```python
from build123d import *

# Parameters (mm, degrees)
SKETCH1_W                    = 812.8
SKETCH1_H                    = 78.232
BOSS_EXTRUDE1_DEPTH          = 3.175
EDGE_FLANGE1_STRIP_W         = 14.224
EDGE_FLANGE1_STRIP_H         = 3.175
EDGE_FLANGE1_STRIP_CUT_DEPTH = 812.8
EDGE_FLANGE1_DEPTH           = 812.8
EDGE_FLANGE2_STRIP_W         = 14.224
EDGE_FLANGE2_STRIP_H         = 3.175
EDGE_FLANGE2_STRIP_CUT_DEPTH = 812.8
EDGE_FLANGE2_DEPTH           = 812.8
SKETCH9_R                    = 2.667
CUT_EXTRUDE1_DEPTH           = 818.620012948
CHAMFER1_SIZE                = 3.175
SKETCH12_R                   = 1.27
CUT_EXTRUDE4_DEPTH           = 818.20071162
SKETCH15_W                   = 812.8
SKETCH15_H                   = 50.8
BOSS_EXTRUDE2_DEPTH          = 3.175
SKETCH16_W                   = 814.386282527
SKETCH16_H                   = 36.576
BOSS_EXTRUDE3_DEPTH          = 3.175


# Sheet-metal steps are written as plain solids
with BuildPart() as part:
    # Sketch1 → Boss-Extrude1 (new body)
    with BuildSketch(Plane(origin=(0, 0, 0), x_dir=(1, 0, 0), z_dir=(0, 1, 0))):
        with Locations((406.4, 39.116)):
            Rectangle(SKETCH1_W, SKETCH1_H)
    extrude(amount=BOSS_EXTRUDE1_DEPTH)

    # Edge-Flange1 strip (across the edge) → Edge-Flange1 strip cut (cut)
    with BuildSketch(Plane(origin=(812.8, 3.175, -78.232), x_dir=(0, 0, 1), z_dir=(-1, 0, 0))):
        with Locations((-6.35, -1.5875)):
            Rectangle(EDGE_FLANGE1_STRIP_W, EDGE_FLANGE1_STRIP_H)
    extrude(amount=EDGE_FLANGE1_STRIP_CUT_DEPTH, mode=Mode.SUBTRACT)

    # Edge-Flange1 section (across the edge) → Edge-Flange1 (add)
    with BuildSketch(Plane(origin=(812.8, 3.175, -78.232), x_dir=(0, 0, 1), z_dir=(-1, 0, 0))):
        with BuildLine():
            Line((-3.175, 0.762), (-3.175, 23.368))
            Line((-3.175, 23.368), (0, 23.368))
            Line((0, 23.368), (0, 0.762))
            ThreePointArc((0, 0.762), (0.223184633, 0.223184633), (0.762, 0))
            Line((0.762, 0), (0.762, -3.175))
            ThreePointArc((0.762, -3.175), (-2.021879398, -2.021879398), (-3.175, 0.762))
        make_face()
    extrude(amount=EDGE_FLANGE1_DEPTH)

    # Edge-Flange2 strip (across the edge) → Edge-Flange2 strip cut (cut)
    with BuildSketch(Plane(origin=(0, 3.175, 0), x_dir=(0, 0, -1), z_dir=(1, 0, 0))):
        with Locations((-6.35, -1.5875)):
            Rectangle(EDGE_FLANGE2_STRIP_W, EDGE_FLANGE2_STRIP_H)
    extrude(amount=EDGE_FLANGE2_STRIP_CUT_DEPTH, mode=Mode.SUBTRACT)

    # Edge-Flange2 section (across the edge) → Edge-Flange2 (add)
    with BuildSketch(Plane(origin=(0, 3.175, 0), x_dir=(0, 0, -1), z_dir=(1, 0, 0))):
        with BuildLine():
            Line((-3.175, 0.762), (-3.175, 23.368))
            Line((-3.175, 23.368), (0, 23.368))
            Line((0, 23.368), (0, 0.762))
            ThreePointArc((0, 0.762), (0.223184633, 0.223184633), (0.762, 0))
            Line((0.762, 0), (0.762, -3.175))
            ThreePointArc((0.762, -3.175), (-2.021879398, -2.021879398), (-3.175, 0.762))
        make_face()
    extrude(amount=EDGE_FLANGE2_DEPTH)

    # Sketch9 → Cut-Extrude1 (cut, through all)
    with BuildSketch(Plane.XY.offset(3.175)):
        with Locations((806.45, 16.637)):
            Circle(SKETCH9_R)
    extrude(amount=-CUT_EXTRUDE1_DEPTH, mode=Mode.SUBTRACT)

    # Chamfer1
    chamfer1_edges = [part.edges().sort_by_distance(p)[0] for p in [
        (812.8, 26.543, -79.8195),
        (0, 26.543, -79.8195),
        (0, 26.543, 1.5875),
        (812.8, 26.543, 1.5875),
    ]]
    chamfer(chamfer1_edges, length=CHAMFER1_SIZE)

    # Sketch12 → Cut-Extrude4 (cut, through all)
    with BuildSketch(Plane(origin=(0, 3.175, 0), x_dir=(1, 0, 0), z_dir=(0, 1, 0))):
        with Locations(Location((127, 72.39, 0), (0, 0, 270))):
            Circle(SKETCH12_R)
        with Locations(Location((228.6, 72.39, 0), (0, 0, 270))):
            Circle(SKETCH12_R)
        with Locations(Location((228.6, 5.842, 0), (0, 0, 270))):
            Circle(SKETCH12_R)
        with Locations(Location((127, 5.842, 0), (0, 0, 270))):
            Circle(SKETCH12_R)
    extrude(amount=-CUT_EXTRUDE4_DEPTH, mode=Mode.SUBTRACT)

    # Sketch15 → Boss-Extrude2 (add)
    with BuildSketch(Plane(origin=(0, 0, -81.407), x_dir=(-1, 0, 0), z_dir=(0, 0, -1))):
        with Locations((-406.4, 25.4)):
            Rectangle(SKETCH15_W, SKETCH15_H)
    extrude(amount=-BOSS_EXTRUDE2_DEPTH)

    # Sketch16 → Boss-Extrude3 (add)
    with BuildSketch(Plane.XY.offset(3.175)):
        with Locations((407.193141264, 18.288)):
            Rectangle(SKETCH16_W, SKETCH16_H)
    extrude(amount=-BOSS_EXTRUDE3_DEPTH)


solid = part.part
```
Verification items for the finished model (mm, model axes). A direction names the side the tool comes from. Coordinates: 2 decimals unless noted, no trailing zeros. Write each loop counter-clockwise with the first axis right and the second up, starting at its lowest first coordinate (ties: lowest second). Pieces come first, ordered by that corner, then holes. Notation, with made-up numbers: M 5,34 L 57,34 A31 cw 57,70 Z; hole C 26.5,66 d3. An arc over 180 degrees is marked long. One line per item, written item: value.
Item 1: Scan lines: line 1 along X through (y, z) = (2.05, -72.39); line 2 along Z through (x, y) = (127, 1.65) (3 decimals); line 3 along X through (y, z) = (2, -72). Record each from-to range of solid material in increasing order.
Check sheet entries:
line 1: x = 0 to 125.73, 128.27 to 227.33, 229.87 to 812.8
line 2: z = -81.407 to -73.66, -71.12 to -7.112, -4.572 to 3.175
line 3: x = 0 to 125.79, 128.21 to 227.39, 229.81 to 812.8
Item 2: Mould release check, pull along Z, two halves, no side actions. Record for faces 1 (the flat face through (401, 19, 3.175)), 2 (the flat face through (0, 3, -39)), 3 (the flat face through (401, 3.175, -40)): pulls with the +Z half, pulls with the -Z half, needs draft (parallel to the pull), parting line crosses it, or undercut.
Check sheet entries:
face 1: pulls with the +Z half
face 2: needs draft
face 3: undercut
Item 3: Section check A-A, the plane y = 10.5. Record the boundary of the cut face in (x, z) (3 decimals), plus the area to 3 significant figures.
Check sheet entries:
outline: M 0,-81.407 L 812.8,-81.407 L 812.8,-78.232 L 0,-78.232 Z; M 0,0 L 814.386,0 L 814.386,3.175 L 0,3.175 Z
area: 5,170 mm^2
Item 4: Section check B-B, the plane x = 142.5. Record the boundary of the cut face in (y, z) (3 decimals).
Check sheet entries:
outline: M 0,-81.407 L 50.8,-81.407 L 50.8,-78.232 L 3.937,-78.232 A0.762 cw 3.175,-77.47 L 3.175,-0.762 A0.762 cw 3.937,0 L 36.576,0 L 36.576,3.175 L 0,3.175 L 0,0 L 0.074,0 A3.937 ccw 0,-0.762 L 0,-77.47 A3.937 ccw 0.074,-78.232 L 0,-78.232 Z
Item 5: Gauge pin test, flat ends, axial feed: pin 1 Ø3 at (x, z) = (228.6, -72.39) entering from -Y; pin 2 Ø6 at (x, z) = (301.5, -29.5) entering from +Y (3 decimals); pin 3 Ø3.5 at (x, z) = (490, 2) entering from +Y. Record the tip position at first contact, or that the pin passes through.
Check sheet entries:
pin 1: stops at y = 0
pin 2: stops at y = 3.175
pin 3: stops at y = 36.58
Item 6: Section check C-C, the plane z = -36. Record the boundary of the cut face in (x, y) (3 decimals).
Check sheet entries:
outline: M 0,0 L 812.8,0 L 812.8,3.175 L 0,3.175 Z
Item 7: Access from +Z, -Z, +X, -X, +Y, -Y to the whole of each face (thin tool, end or side, straight path). Record for faces 4 (the flat face through (412, 28, -78.232)), 5 (the flat face through (412, 26, -81.407)), 6 (the flat face through (812.8, 3, -53)).
Check sheet entries:
face 4: +X, -X, +Y
face 5: -Z, +X, -X, +Y, -Y
face 6: -Z, +X, +Y, -Y
